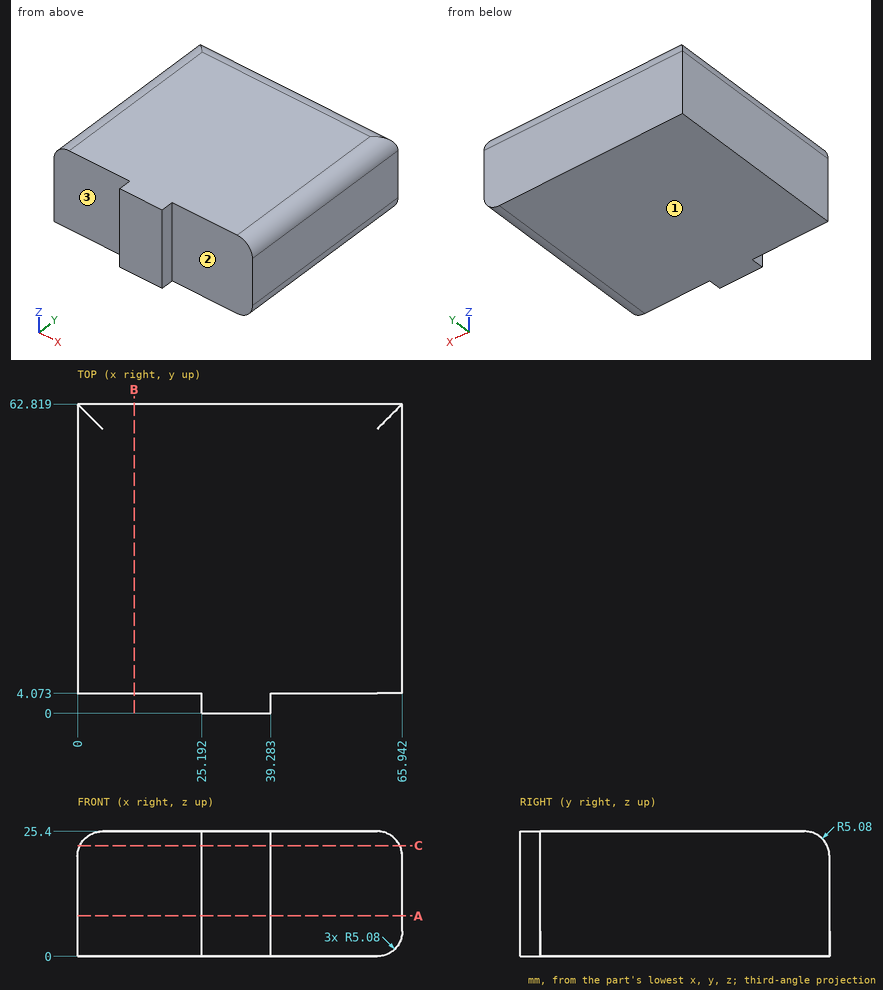
The figure shows three views and two pictorial views of one solid part (mm, origin at its lowest corner). Answer the questions. A direction names the side the tool comes from. Give positions to 0.01 mm unless a question says otherwise; leave off trailing zeros. Write each loop counter-clockwise with the first axis right and the second up, starting at its lowest first coordinate (ties: lowest second). Pieces come first, ordered by that corner, then holes. Notation, with made-up numbers: (44, 88) - (94, 88) arc R18 cw to (94, 110) - close; hole circle Ø7 at (33.5, 29). An arc over 180 degrees is marked (long way). Return JSON: item names as keys, results as strings.
Q1. Consider line 1 along Y through (x, z) = (42, 15.5); line 2 along Z through (x, y) = (8, 58); line 3 along X through (y, z) = (42.5, 2.75) (1 decimal). Determine where each line is inside the solid, lowest interval first. Write a range as [from, to].
Reply:
{"line 1": "[4.07, 62.82]", "line 2": "[0, 25.39]", "line 3": "[0, 65.4]"}
Q2. For the marked faces 1, 2 and 3, determine the directions among +Z, -Z, +X, -X, +Y, -Y from which every point of the face is accessible in a straight line to the end or side of a thin tool.
Reply:
{"face 1": "-Z, +X, -X, +Y, -Y", "face 2": "+Z, -Z, +X, -Y", "face 3": "+Z, -Z, -X, -Y"}
Q3. A cutting plane is placed at A-A, the plane z = 8.25. Determine the outline of the cut face in (x, y), and give its area (3 significant figures).
Reply:
{"outline": "(0, 4.07) - (25.19, 4.07) - (25.19, 0) - (39.28, 0) - (39.28, 4.07) - (65.94, 4.07) - (65.94, 62.82) - (0, 62.82) - close", "area": "3,930 mm²"}
Q4. A cutting plane is placed at C-C, the plane z = 22.5. Determine the outline of the cut face in (x, y), and give its area (3 significant figures).
Reply:
{"outline": "(0.49, 4.07) - (25.19, 4.07) - (25.19, 0) - (39.28, 0) - (39.28, 4.07) - (65.45, 4.07) - (65.45, 62.33) - (0.49, 62.33) - close", "area": "3,840 mm²"}
Q5. Given P1, Ø1.2, axis at y = 1.5, z = 7, coming from the -X side; P2, Ø12, axis at x = 45.5, z = 3, coming from the -Y side; P3, Ø4.5, axis at y = 1.5, z = 15.5, coming from the +X side, each flat-ended and moving along its own axis, determine where each tip first touches the part or whether it passes through.
Reply:
{"P1": "x = 25.19", "P2": "y = 4.07", "P3": "x = 39.28"}
Q6. A cutting plane is placed at B-B, the plane x = 11.5. Determine the outline of the cut face in (y, z), and give its area (3 significant figures).
Reply:
{"outline": "(4.07, 0) - (62.82, 0) - (62.82, 20.32) arc R5.08 ccw to (57.74, 25.4) - (4.07, 25.4) - close", "area": "1,490 mm²"}
